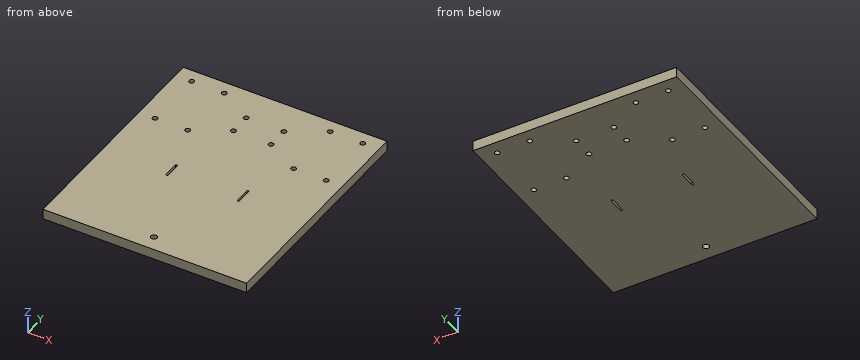
```python
from build123d import *

# Parameters (mm, degrees)
SKETCH_W   = 200
SKETCH_H   = 230
SKETCH_R   = 3
SKETCH_R_2 = 2.5
PAD_DEPTH  = 10


with BuildPart() as part:
    # Sketch → Pad (new body)
    with BuildSketch(Plane.XY):
        with Locations((0, 115)):
            Rectangle(SKETCH_W, SKETCH_H)
        with Locations((0, 15)):
            Circle(SKETCH_R, mode=Mode.SUBTRACT)
        with Locations((84, 217)):
            Circle(SKETCH_R_2, mode=Mode.SUBTRACT)
        with Locations((84, 157)):
            Circle(SKETCH_R_2, mode=Mode.SUBTRACT)
        with Locations((52, 157)):
            Circle(SKETCH_R_2, mode=Mode.SUBTRACT)
        with Locations((52, 217)):
            Circle(SKETCH_R_2, mode=Mode.SUBTRACT)
        with Locations((-84, 217)):
            Circle(SKETCH_R_2, mode=Mode.SUBTRACT)
        with Locations((-52, 217)):
            Circle(SKETCH_R_2, mode=Mode.SUBTRACT)
        with Locations((-84, 157)):
            Circle(SKETCH_R_2, mode=Mode.SUBTRACT)
        with Locations((-52, 157)):
            Circle(SKETCH_R_2, mode=Mode.SUBTRACT)
        with Locations((-18.5, 197)):
            Circle(SKETCH_R_2, mode=Mode.SUBTRACT)
        with Locations((18.5, 197)):
            Circle(SKETCH_R_2, mode=Mode.SUBTRACT)
        with Locations((-18.5, 176)):
            Circle(SKETCH_R_2, mode=Mode.SUBTRACT)
        with Locations((18.5, 176)):
            Circle(SKETCH_R_2, mode=Mode.SUBTRACT)
        with BuildLine():
            ThreePointArc((36, 110), (35, 111), (34, 110))
            Line((34, 110), (34, 95))
            ThreePointArc((34, 95), (35, 94), (36, 95))
            Line((36, 110), (36, 95))
        make_face(mode=Mode.SUBTRACT)
        with BuildLine():
            ThreePointArc((-34, 109.999637), (-35, 110.999637), (-36, 109.999637))
            Line((-36, 109.999637), (-36, 95))
            ThreePointArc((-36, 95), (-35, 94), (-34, 95))
            Line((-34, 109.999637), (-34, 95))
        make_face(mode=Mode.SUBTRACT)
    extrude(amount=PAD_DEPTH)


solid = part.part
```
Could you check a few things on this model? Use its own coordinates, in mm. Round coordinates to 2 decimals unless told otherwise and drop trailing zeros. Loops run counter-clockwise (first coordinate to the right, second up) from the corner with the lowest first, then second, coordinate; pieces in that order, holes last.
Q1. I want a section at C-C (y = 103). Write out the boundary of the cut face in (x, z), and give its area (3 significant figures).
Q2. I want a section at D-D (x = 0). Write out the boundary of the cut face in (y, z), and give its area (3 significant figures).
Q3. For P1, Ø3, axis at x = 84, y = 157, coming from the -Z side, with a flat end and sliding along its axis, tell me the tip position at first contact or that it passes through.
Q4. I want a section at B-B (y = 15). Write out the boundary of the cut face in (x, z), and give its area (3 significant figures).
Q5. I want a section at A-A (x = -52). Write out the boundary of the cut face in (y, z), and give its area (3 significant figures).
Q6. Please list where these lines run through material, in increasing order: L1, parallel to X at y = 101, z = 8.5; L2, parallel to X at y = 176, z = 4; L3, parallel to Y at x = 18.5, z = 4.
Answer below:
1. outline: (-100, 0) - (-36, 0) - (-36, 10) - (-100, 10) - close; (-34, 0) - (34, 0) - (34, 10) - (-34, 10) - close; (36, 0) - (100, 0) - (100, 10) - (36, 10) - close
1. area: 1,960 mm2
2. outline: (0, 0) - (12, 0) - (12, 10) - (0, 10) - close; (18, 0) - (230, 0) - (230, 10) - (18, 10) - close
2. area: 2,240 mm2
3. P1: passes through
4. outline: (-100, 0) - (-3, 0) - (-3, 10) - (-100, 10) - close; (3, 0) - (100, 0) - (100, 10) - (3, 10) - close
4. area: 1,940 mm2
5. outline: (0, 0) - (154.5, 0) - (154.5, 10) - (0, 10) - close; (159.5, 0) - (214.5, 0) - (214.5, 10) - (159.5, 10) - close; (219.5, 0) - (230, 0) - (230, 10) - (219.5, 10) - close
5. area: 2,200 mm2
6. L1: x = -100 to -36, -34 to 34, 36 to 100
6. L2: x = -100 to -21, -16 to 16, 21 to 100
6. L3: y = 0 to 173.5, 178.5 to 194.5, 199.5 to 230
